Could you check a few things on this drawing? It's one solid part, dimensions in mm from its lowest x, y, z. Coordinates: 2 decimals unless noted, no trailing zeros. Write each loop counter-clockwise with the first axis right and the second up, starting at its lowest first coordinate (ties: lowest second). Pieces come first, ordered by that corner, then holes. Notation, with made-up numbers: (37, -12.75) - (69, -12.75) arc R23 ccw to (69, 2.25) - close; hole circle Ø1 at (76.25, 5). An arc over 180 degrees is marked (long way). Answer as a JSON object with one key per item and string values. Group by question number.
1) If we section it at A-A (x = 575): Write out the boundary of the cut face in (y, z).
2) If we section it at D-D (z = 396): Write out the boundary of the cut face in (x, y).
3) If we section it at B-B (z = 231): Write out the boundary of the cut face in (x, y), plus the area to 3 significant figures.
4) Please list where these lines run through material, in increasing order: line 1 along Z through (x, y) = (530.5, 19); line 2 along Y through (x, z) = (197.5, 262.5); line 3 along X through (y, z) = (16, 163.5).
5) If we section it at C-C (y = 12.5): Write out the boundary of the cut face in (x, z), plus the area to 3 significant figures.
6) Will these pins go through, and if not, where does the flat tip stop? pin 1 Ø9 at (x, y) = (1080, 42) entering from -Z; pin 2 Ø3 at (y, z) = (15, 233) entering from +X; pin 3 Ø24 at (x, y) = (589, 11.5) entering from -Z; pin 4 Ø1 at (x, z) = (729, 200) entering from -Y.
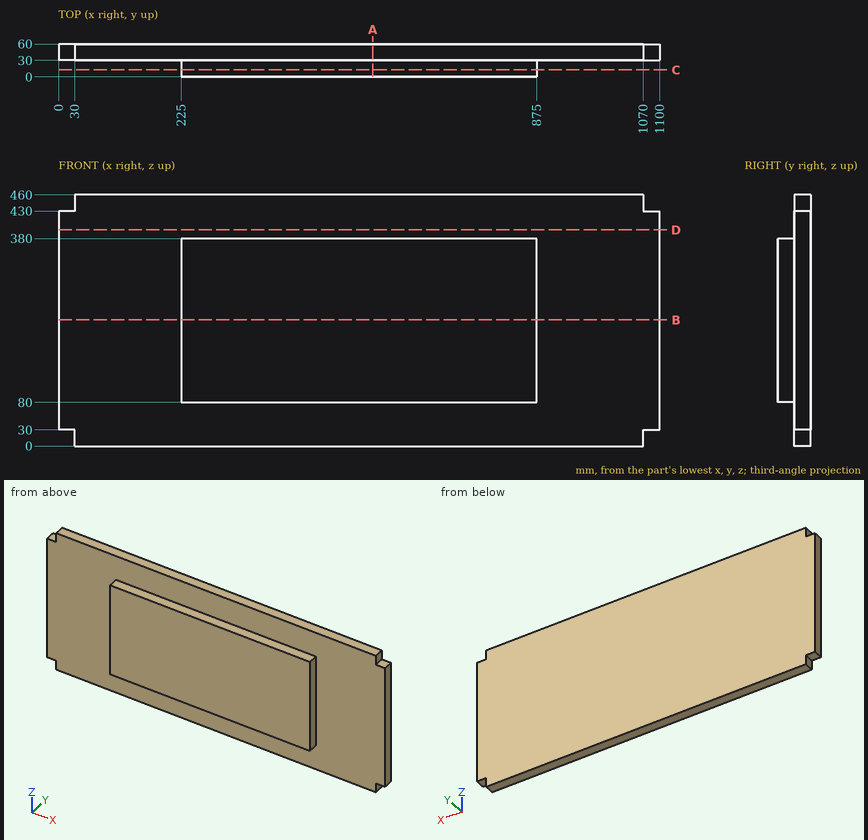
Here are the results:
{
 "1": {"outline": "(0, 80) - (30, 80) - (30, 0) - (60, 0) - (60, 460) - (30, 460) - (30, 380) - (0, 380) - close"},
 "2": {"outline": "(0, 30) - (1100, 30) - (1100, 60) - (0, 60) - close"},
 "3": {"outline": "(0, 30) - (225, 30) - (225, 0) - (875, 0) - (875, 30) - (1100, 30) - (1100, 60) - (0, 60) - close", "area": "52,500 mm²"},
 "4": {"line 1": "z = 80 to 380", "line 2": "y = 30 to 60", "line 3": "x = 225 to 875"},
 "5": {"outline": "(225, 80) - (875, 80) - (875, 380) - (225, 380) - close", "area": "195,000 mm²"},
 "6": {"pin 1": "stops at z = 30", "pin 2": "stops at x = 875", "pin 3": "stops at z = 80", "pin 4": "stops at y = 0"}
}
